Geometry check sheet. Reference: the model listing, model coordinates, mm. Coordinates: 2 decimals unless noted, no trailing zeros. Loops run counter-clockwise (first coordinate to the right, second up) from the corner with the lowest first, then second, coordinate; pieces in that order, holes last.
from build123d import *

# Parameters (mm, degrees)
SKETCH2_R           = 35
SKETCH2_W           = 100
SKETCH2_H           = 4
BOSS_EXTRUDE1_DEPTH = 4


with BuildPart() as part:
    # Sketch2 → Boss-Extrude1 (new body)
    with BuildSketch(Plane(origin=(0, 0, 0), x_dir=(1, 0, 0), z_dir=(0, 1, 0))):
        Polygon((-50, 84), (50, 84), (50, 80), (91, 80), (91, 70), (95, 70), (95, 50), (91, 50), (91, -108), (95, -108), (95, -128), (91, -128), (91, -138), (-91, -138), (-91, -128), (-95, -128), (-95, -108), (-91, -108), (-91, 50), (-95, 50), (-95, 70), (-91, 70), (-91, 80), (-50, 80), align=None)
        with Locations((0, 40.261243559)):
            Circle(SKETCH2_R, mode=Mode.SUBTRACT)
        with Locations((0, -82.68297303)):
            Circle(SKETCH2_R, mode=Mode.SUBTRACT)
        with Locations((0, -29)):
            Rectangle(SKETCH2_W, SKETCH2_H, mode=Mode.SUBTRACT)
    extrude(amount=BOSS_EXTRUDE1_DEPTH)


solid = part.part
1) Section check A-A on x = 0. Record the cut outline in (y, z), and give its area (3 significant figures).
Data:
outline: (0, -84) - (4, -84) - (4, -75.26) - (0, -75.26) - close; (0, -5.26) - (4, -5.26) - (4, 27) - (0, 27) - close; (0, 31) - (4, 31) - (4, 47.68) - (0, 47.68) - close; (0, 117.68) - (4, 117.68) - (4, 138) - (0, 138) - close
area: 312 mm2
2) Section check D-D on x = -60. Record the cut outline in (y, z).
Data:
outline: (0, -80) - (4, -80) - (4, 138) - (0, 138) - close
3) Section check B-B on y = 3.3. Count the separate pieces of the cut face and the enclosed holes in it, and give its area (3 significant figures).
Data:
separate pieces: 1
enclosed holes: 3
area: 32,300 mm2
4) Mould release check, pull along X, two halves, no side actions. Record for faces 1 (the cylindrical face through (-7.59, 1.97, 116.85)), 2 (the flat face through (1, 0, 25)): +X half, -X half, draft (parallel to the pull), parting line (faces both ways), or undercut.
Data:
face 1: undercut
face 2: draft
5) Section check C-C on z = 112. Record the cut outline in (x, y).
Data:
outline: (-95, 0) - (-19.12, 0) - (-19.12, 4) - (-95, 4) - close; (19.12, 0) - (95, 0) - (95, 4) - (19.12, 4) - close
6) Depth check by flat-ended pin: pin 1 (2 mm diameter, centred on y = 2, z = 132.5, fed in from -X); pin 2 (1.2 mm diameter, centred on y = 2, z = -77, fed in from +X); pin 3 (1.2 mm diameter, centred on x = 92, y = 3, fed in from +Z). Enter the tip coordinate at first touch or a pass-through.
Data:
pin 1: stops at x = -91
pin 2: stops at x = 91
pin 3: stops at z = 128
7) Material ranges on probe 1 along Z at (x, y) = (0, 1.3); probe 2 along Z at (x, y) = (30, 2.9); probe 3 along X at (y, z) = (1.6, -42), recorded low to high.
Data:
probe 1: z = -84 to -75.26, -5.26 to 27, 31 to 47.68, 117.68 to 138
probe 2: z = -84 to -58.29, -22.23 to 27, 31 to 64.66, 100.71 to 138
probe 3: x = -91 to -34.96, 34.96 to 91
